Geometry check sheet. Reference: drawing and pictorial views, mm from the part's lowest x, y, z. A direction names the side the tool comes from. Give positions to 0.01 mm unless a question says otherwise; leave off trailing zeros. Order: outer loops, then holes, each group sorted by start corner. A loop starts at its lowest first (then second) coordinate and runs counter-clockwise, first axis right, second up. Notation, with made-up numbers: (-9.75, 13.25) - (-0.75, 13.25) arc R16 ccw to (-0.75, 23.25) - close; hole circle Ø7 at (73, -3.75). An arc over 180 degrees is marked (long way). Answer in a Markdown table with one row per item.
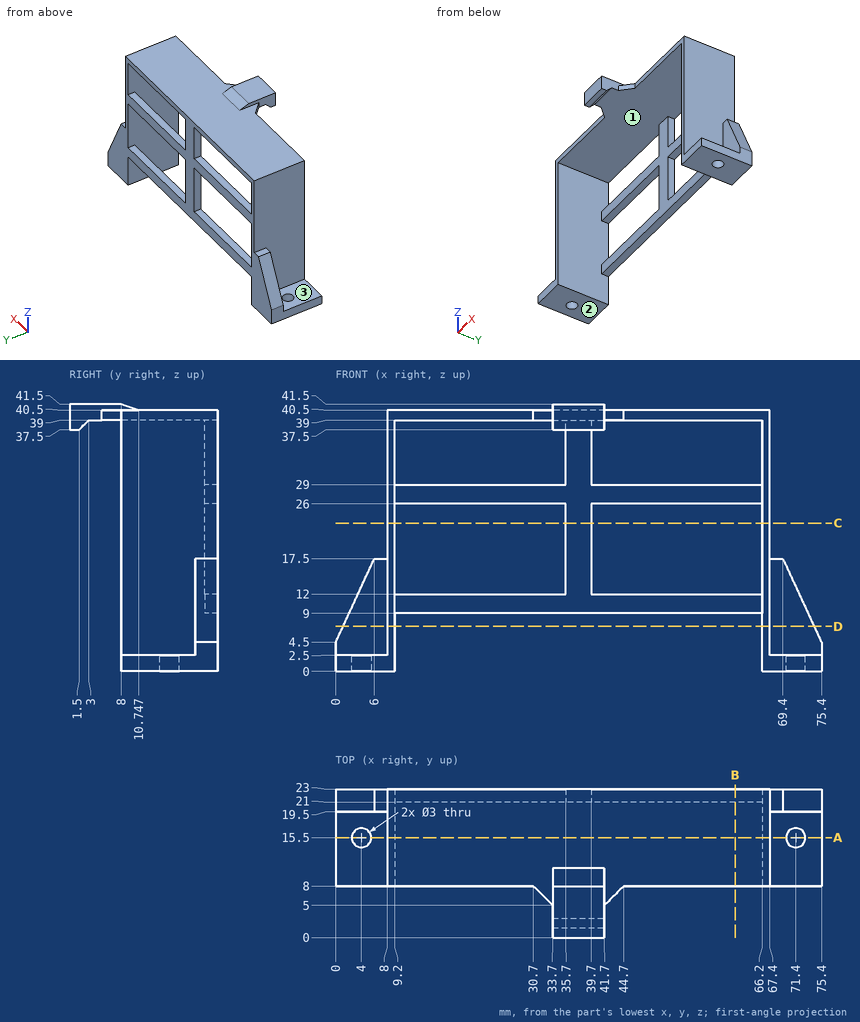
(1) Cross-section at D-D, the plane z = 7. Record the cut outline in (x, y).
Geometry says:
| item | result |
|---|---|
| outline | (1.15, 19.5) - (8, 19.5) - (8, 8) - (9.2, 8) - (9.2, 23) - (1.15, 23) - close; (66.2, 8) - (67.4, 8) - (67.4, 19.5) - (74.25, 19.5) - (74.25, 23) - (66.2, 23) - close |
(2) Cross-section at A-A, the plane y = 15.5. Record the cut outline in (x, z).
Geometry says:
| item | result |
|---|---|
| outline | (0, 0) - (2.5, 0) - (2.5, 2.5) - (0, 2.5) - close; (5.5, 0) - (9.2, 0) - (9.2, 39) - (66.2, 39) - (66.2, 0) - (69.9, 0) - (69.9, 2.5) - (67.4, 2.5) - (67.4, 40.5) - (8, 40.5) - (8, 2.5) - (5.5, 2.5) - close; (72.9, 0) - (75.4, 0) - (75.4, 2.5) - (72.9, 2.5) - close |
(3) Gauge pin test, flat ends, axial feed: P1, Ø1.5, axis at x = 37, z = 20.5, coming from the -Y side; P2, Ø3, axis at y = 9, z = 17.5, coming from the +X side; P3, Ø0.6, axis at x = 68, y = 20.5, coming from the +Z side; P4, Ø9, axis at x = 31, z = 21, coming from the -Y side. Record the tip position at first contact, or that the pin passes through.
Geometry says:
| item | result |
|---|---|
| P1 | y = 21 |
| P2 | x = 67.4 |
| P3 | z = 17.5 |
| P4 | through |
(4) Access from +Z, -Z, +X, -X, +Y, -Y to the whole of each face (thin tool, end or side, straight path). Record for the marked faces 1, 2 and 3.
Geometry says:
| item | result |
|---|---|
| face 1 | none |
| face 2 | -Z, +X, -X, +Y, -Y |
| face 3 | +Z, -X, -Y |
(5) Thickness scan on L1, parallel to Z at x = 62.5, y = 21.25; L2, parallel to Y at x = 4, z = 1; L3, parallel to X at y = 12.5, z = 13. Record the ranges inside material, lowest first.
Geometry says:
| item | result |
|---|---|
| L1 | 9 to 12, 26 to 29, 39 to 40.5 |
| L2 | 8 to 14, 17 to 23 |
| L3 | 8 to 9.2, 66.2 to 67.4 |
(6) Cross-section at B-B, the plane x = 62. Record the cut outline in (y, z).
Geometry says:
| item | result |
|---|---|
| outline | (8, 39) - (23, 39) - (23, 40.5) - (8, 40.5) - close; (21, 9) - (23, 9) - (23, 12) - (21, 12) - close; (21, 26) - (23, 26) - (23, 29) - (21, 29) - close |
(7) Cross-section at C-C, the plane z = 23. Record the cut outline in (x, y).
Geometry says:
| item | result |
|---|---|
| outline | (8, 8) - (9.2, 8) - (9.2, 23) - (8, 23) - close; (35.7, 21) - (39.7, 21) - (39.7, 23) - (35.7, 23) - close; (66.2, 8) - (67.4, 8) - (67.4, 23) - (66.2, 23) - close |
